Here's how the part is built. I have some questions about the finished solid (model axes, mm). Face numbers are marked on the shaded views. A direction names the side the tool comes from. Coordinates: 2 decimals unless noted, no trailing zeros. Write each loop counter-clockwise with the first axis right and the second up, starting at its lowest first coordinate (ties: lowest second). Pieces come first, ordered by that corner, then holes.
Item 1: I'm going to push flat-ended pins straight in: pin 1 Ø4 at (x, z) = (-145.5, 16.5) entering from +Y; pin 2 Ø1 at (y, z) = (-69, 50) entering from -X (3 decimals); pin 3 Ø1.5 at (x, y) = (-42, -43) entering from -Z. Where does each tip first touch, or does it pass through?
Item 2: If we section it at D-D (z = 82): Please give me the cut outline in (x, y) (3 decimals).
Item 3: If I drill on line 1 (Y direction, x = -10, z = 97); line 2 (X direction, y = -143, z = 72.5) (3 decimals); line 3 (Y direction, x = -142, z = 75.5), over which ranges is the centre line in solid material (lowest first)?
Item 4: If we section it at B-B (x = 91.5): Please give me the cut outline in (y, z).
Item 5: We'd pull the mould along X, two halves only. Please class the marked faces 3, 4 and 5: +X half, -X half, draft (parallel to the pull), parting line (faces both ways), or undercut.
Item 6: If we section it at C-C (y = 143.5): Please give me the cut outline in (x, z) (3 decimals).
Item 7: If we section it at A-A (z = 299): Please give me the cut outline in (x, y) (3 decimals).
Item 8: For the marked faces 1 and 2, which set-ups out of +Z, -Z, +X, -X, +Y, -Y let a thin tool reach every point of the face, with its end or its side?
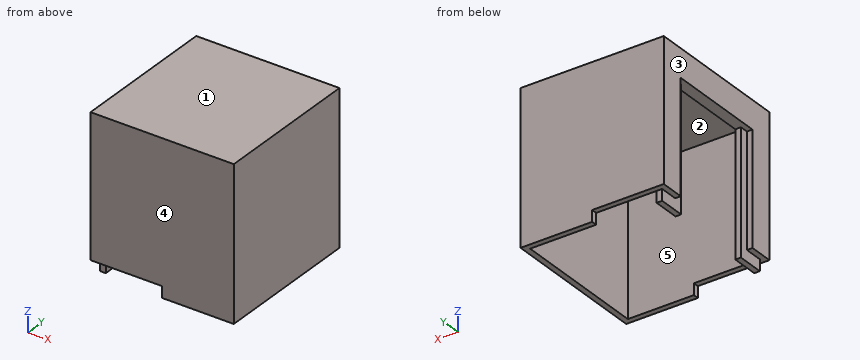
from build123d import *

# Parameters (mm, degrees)
F0_W      = 161.925
F0_H      = 336.55
F1_DEPTH  = 342.9
F2_W      = 285.75
F2_H      = 311.15
F3_DEPTH  = 317.5
F4_W      = 165.1
F4_H      = 222.25
F5_DEPTH  = 50.8
F6_W      = 228.6
F6_H      = 279.4
F7_DEPTH  = 76.2
F8_W      = 355.6
F8_H      = 25.4
F9_DEPTH  = 203.2
F10_W     = 12.7
F10_H     = 254
F12_DEPTH = 19.05
F13_W     = 12.7
F13_H     = 254
F14_DEPTH = 19.05
F15_W     = 12.7
F15_H     = 60.325
F16_DEPTH = 25.4
F17_W     = 12.7
F17_H     = 60.325
F18_DEPTH = 25.4


with BuildPart() as f1:
    # F0 (on Top) → F1 (new body)
    with BuildSketch(Plane.XY):
        with Locations((-80.9625, 4.714677)):
            Rectangle(F0_W, F0_H)
        with Locations((80.9625, 4.714677)):
            Rectangle(F0_W, F0_H)
    extrude(amount=F1_DEPTH)

    # F2 (on face) → F3 (cut)
    with BuildSketch(Plane(origin=(0, 0, 0), x_dir=(1, 0, 0), z_dir=(0, 0, -1))):
        with Locations((6.35, -4.714677)):
            Rectangle(F2_W, F2_H)
    extrude(amount=-F3_DEPTH, mode=Mode.SUBTRACT)

    # F4 (on face) → F5 (cut)
    with BuildSketch(Plane(origin=(-161.925, 0, 0), x_dir=(0, -1, 0), z_dir=(-1, 0, 0))):
        with Locations((-4.714677, 111.125)):
            Rectangle(F4_W, F4_H)
    extrude(amount=-F5_DEPTH, mode=Mode.SUBTRACT)

    # F6 (on face) → F7 (cut)
    with BuildSketch(Plane(origin=(-161.925, 0, 0), x_dir=(0, -1, 0), z_dir=(-1, 0, 0))):
        with Locations((-4.714677, 139.7)):
            Rectangle(F6_W, F6_H)
    extrude(amount=-F7_DEPTH, mode=Mode.SUBTRACT)

    # F8 (on Right) → F9 (cut)
    with BuildSketch(Plane.YZ):
        with Locations((5.509312, 12.7)):
            Rectangle(F8_W, F8_H)
    extrude(amount=-F9_DEPTH, mode=Mode.SUBTRACT)

    # F10 (on face) → F12 (join)
    with BuildSketch(Plane.XZ.offset(-119.014677)):
        with Locations((-142.875, 152.4)):
            Rectangle(F10_W, F10_H)
    extrude(amount=F12_DEPTH)

    # F13 (on face) → F14 (join)
    with BuildSketch(Plane(origin=(0, -109.585323, 0), x_dir=(-1, 0, 0), z_dir=(0, 1, 0))):
        with Locations((142.875, 152.4)):
            Rectangle(F13_W, F13_H)
    extrude(amount=F14_DEPTH)

    # F15 (on face) → F16 (join)
    with BuildSketch(Plane(origin=(0, 0, 25.4), x_dir=(1, 0, 0), z_dir=(0, 0, -1))):
        with Locations((-142.875, 120.697823)):
            Rectangle(F15_W, F15_H)
    extrude(amount=F16_DEPTH)

    # F17 (on face) → F18 (join)
    with BuildSketch(Plane(origin=(0, 0, 25.4), x_dir=(1, 0, 0), z_dir=(0, 0, -1))):
        with Locations((-142.875, -130.127177)):
            Rectangle(F17_W, F17_H)
    extrude(amount=F18_DEPTH)


solid = f1.part
Answer list:
1. pin 1: stops at y = 160.29
1. pin 2: stops at x = 149.225
1. pin 3: stops at z = 317.5
2. outline: (-161.925, -163.56) - (161.925, -163.56) - (161.925, 172.99) - (-161.925, 172.99) - (-161.925, 119.015) - (-149.225, 119.015) - (-149.225, 99.965) - (-136.525, 99.965) - (-136.525, 160.29) - (149.225, 160.29) - (149.225, -150.86) - (-136.525, -150.86) - (-136.525, -90.535) - (-149.225, -90.535) - (-149.225, -109.585) - (-161.925, -109.585) - close
3. line 1: y = -163.56 to -150.86, 160.29 to 172.99
3. line 2: x = -161.925 to -136.525, 149.225 to 161.925
3. line 3: y = -163.56 to -90.54, 99.96 to 172.99
4. outline: (-163.56, 0) - (-150.86, 0) - (-150.86, 317.5) - (160.29, 317.5) - (160.29, 0) - (172.99, 0) - (172.99, 342.9) - (-163.56, 342.9) - close
5. face 3: -X half
5. face 4: draft
5. face 5: undercut
6. outline: (-161.925, 25.4) - (-149.225, 25.4) - (-149.225, 0) - (-136.525, 0) - (-136.525, 317.5) - (149.225, 317.5) - (149.225, 0) - (161.925, 0) - (161.925, 342.9) - (-161.925, 342.9) - close
7. outline: (-161.925, -163.56) - (161.925, -163.56) - (161.925, 172.99) - (-161.925, 172.99) - close; hole (-136.525, -150.86) - (149.225, -150.86) - (149.225, 160.29) - (-136.525, 160.29) - close
8. face 1: +Z, +X, -X, +Y, -Y
8. face 2: -Z
